Build history of the part. All positions in model axes, mm. A direction names the side the tool comes from. Coordinates: 2 decimals unless noted, no trailing zeros. Order: outer loops, then holes, each group sorted by start corner. A loop starts at its lowest first (then second) coordinate and runs counter-clockwise, first axis right, second up. Notation, with made-up numbers: (5.25, 60) - (12.25, 60) arc R16 cw to (12.25, 87) - close; hole circle Ø9 at (-25, 15). An arc over 180 degrees is marked (long way). One line per item, written item: value.
from build123d import *

# Parameters (mm, degrees)
F1_DEPTH = 3.5
F2_DEPTH = 150
F3_R     = 5
F4_R     = 1


with BuildPart() as f1:
    # F0 (on Front) → F1 (new body)
    with BuildSketch(Plane.XZ):
        with BuildLine():
            ThreePointArc((3.5, 8.5), (4.9644660941, 4.9644660941), (8.5, 3.5))
            Line((8.5, 3.5), (46.5, 3.5))
            ThreePointArc((46.5, 3.5), (50.0355339059, 4.9644660941), (51.5, 8.5))
            Line((51.5, 8.5), (51.5, 29.5))
            ThreePointArc((51.5, 29.5), (50.0355339059, 33.0355339059), (46.5, 34.5))
            Line((46.5, 34.5), (8.5, 34.5))
            ThreePointArc((8.5, 34.5), (4.9644660941, 33.0355339059), (3.5, 29.5))
            Line((3.5, 29.5), (3.5, 8.5))
        make_face()
    extrude(amount=-F1_DEPTH)

    # F0 (on Front) → F2 (join)
    with BuildSketch(Plane.XZ):
        with BuildLine():
            ThreePointArc((0, 5), (1.4644660941, 1.4644660941), (5, 0))
            Line((5, 0), (50, 0))
            ThreePointArc((50, 0), (53.5355339059, 1.4644660941), (55, 5))
            Line((55, 5), (55, 33))
            ThreePointArc((55, 33), (53.5355339059, 36.5355339059), (50, 38))
            Line((50, 38), (5, 38))
            ThreePointArc((5, 38), (1.4644660941, 36.5355339059), (0, 33))
            Line((0, 33), (0, 5))
        make_face()
        with BuildLine():
            Line((46.5, 3.5), (8.5, 3.5))
            ThreePointArc((8.5, 3.5), (4.9644660941, 4.9644660941), (3.5, 8.5))
            Line((3.5, 8.5), (3.5, 29.5))
            ThreePointArc((3.5, 29.5), (4.9644660941, 33.0355339059), (8.5, 34.5))
            Line((8.5, 34.5), (46.5, 34.5))
            ThreePointArc((46.5, 34.5), (50.0355339059, 33.0355339059), (51.5, 29.5))
            Line((51.5, 29.5), (51.5, 8.5))
            ThreePointArc((51.5, 8.5), (50.0355339059, 4.9644660941), (46.5, 3.5))
        make_face(mode=Mode.SUBTRACT)
    extrude(amount=-F2_DEPTH)

    # F3
    f3_edges = [f1.edges().sort_by_distance(p)[0] for p in [
        (1.464466, 0, 36.535534),
        (0, 0, 19),
        (27.5, 0, 38),
        (53.535534, 0, 36.535534),
        (55, 0, 19),
        (53.535534, 0, 1.464466),
        (27.5, 0, 0),
        (1.464466, 0, 1.464466),
    ]]
    fillet(f3_edges, radius=F3_R)

    # F4
    f4_edges = [f1.edges().sort_by_distance(p)[0] for p in [
        (27.5, 150, 38),
        (53.535534, 150, 36.535534),
        (55, 150, 19),
        (53.535534, 150, 1.464466),
        (27.5, 150, 0),
        (1.464466, 150, 1.464466),
        (0, 150, 19),
        (1.464466, 150, 36.535534),
        (3.5, 150, 19),
        (4.964466, 150, 33.035534),
        (27.5, 150, 34.5),
        (50.035534, 150, 33.035534),
        (51.5, 150, 19),
        (50.035534, 150, 4.964466),
        (27.5, 150, 3.5),
        (4.964466, 150, 4.964466),
    ]]
    fillet(f4_edges, radius=F4_R)


solid = f1.part
1. Probe line 1 along Z through (x, y) = (10, 59); line 2 along X through (y, z) = (51, 29); line 3 along Y through (x, z) = (37, 14). List the from-to ranges inside material, lowest first.
Values found:
line 1: z = 0 to 3.5, 34.5 to 38
line 2: x = 0 to 3.5, 51.5 to 55
line 3: y = 0 to 3.5
2. Band-saw the part on A-A, the plane y = 13.5. Give the cut face in (x, z), and give its area (3 significant figures).
Values found:
outline: (0, 5) arc R5 ccw to (5, 0) - (50, 0) arc R5 ccw to (55, 5) - (55, 33) arc R5 ccw to (50, 38) - (5, 38) arc R5 ccw to (0, 33) - close; hole (3.5, 8.5) arc R5 ccw to (8.5, 3.5) - (46.5, 3.5) arc R5 ccw to (51.5, 8.5) - (51.5, 29.5) arc R5 ccw to (46.5, 34.5) - (8.5, 34.5) arc R5 ccw to (3.5, 29.5) - close
area: 602 mm2
3. Band-saw the part on B-B, the plane x = 14. Give the cut face in (y, z).
Values found:
outline: (0, 5) arc R5 ccw to (5, 0) - (149, 0) arc R1 ccw to (150, 1) - (150, 2.5) arc R1 ccw to (149, 3.5) - (3.5, 3.5) - (3.5, 34.5) - (149, 34.5) arc R1 ccw to (150, 35.5) - (150, 37) arc R1 ccw to (149, 38) - (5, 38) arc R5 ccw to (0, 33) - close
4. Flat gauge pin, fed straight in: P1, Ø9.5, axis at x = 20.5, z = 11.5, coming from the +Y side. Where does the tip first touch, or does it go through?
Values found:
P1: stops at y = 3.5
5. Band-saw the part on C-C, the plane z = 24. Give the cut face in (x, y).
Values found:
outline: (0, 5) arc R5 ccw to (5, 0) - (50, 0) arc R5 ccw to (55, 5) - (55, 149) arc R1 ccw to (54, 150) - (52.5, 150) arc R1 ccw to (51.5, 149) - (51.5, 3.5) - (3.5, 3.5) - (3.5, 149) arc R1 ccw to (2.5, 150) - (1, 150) arc R1 ccw to (0, 149) - close
6. 3-axis set-ups, long thin cutter, end or side, ignore diameter. For faces 1 (the face through (28, 76, 38)), 2 (the face through (50, 75.23, 33.07)): which of +Z, -Z, +X, -X, +Y, -Y reach the whole face in a straight line?
Values found:
face 1: +Z, +X, -X, +Y, -Y
face 2: +Y
